Print and shaded views of the part. All mm, measured from the part's lowest x, y and z. A direction names the side the tool comes from. Round coordinates to 2 decimals unless told otherwise and drop trailing zeros. Order: outer loops, then holes, each group sorted by start corner. A loop starts at its lowest first (then second) coordinate and runs counter-clockwise, first axis right, second up. Notation, with made-up numbers: M 62.5,-28 L 94.5,-28 A14 ccw 94.5,-2 Z; hole C 26.5,13 d3. An arc over 180 degrees is marked long. Write each question's results on one line, items separated by ' | '. Start each with the question number.
1. Probe L1, parallel to X at y = 1.5, z = 9.75; L2, parallel to Y at x = 62.5, z = 9.5; L3, parallel to Y at x = 62.5, z = 17.75. List the from-to ranges inside material, lowest first. Write a range as [from, to].
2. Which spindle directions (+Z, -Z, +X, -X, +Y, -Y) get a long thin tool onto all of the face, cutting with end or side? Do the marked faces 4, 5 and 6. Say none if no direction does.
3. Drop flat-ended pins along their axis: pin 1 Ø3 at (x, z) = (30.5, 6.5) entering from -Y; pin 2 Ø2 at (y, z) = (11.5, 17.5) entering from -X; pin 3 Ø12 at (x, y) = (45.5, 4.5) entering from -Z. Give the stop position or say it passes through.
4. Band-saw the part on B-B, the plane y = 1. List the corners of the cut face in (x, z), then the cut area to 3 significant figures.
5. Band-saw the part on C-C, the plane x = 76. List the corners of the cut face in (y, z), then the cut area to 3 significant figures.
6. Two-plate mould, pull along X, no slides. Class the marked faces 1, 2 and 3: +X half, -X half, draft (parallel to the pull), parting line (faces both ways), or undercut.
7. Band-saw the part on A-A, the plane z = 17. List the corners of the cut face in (x, y).
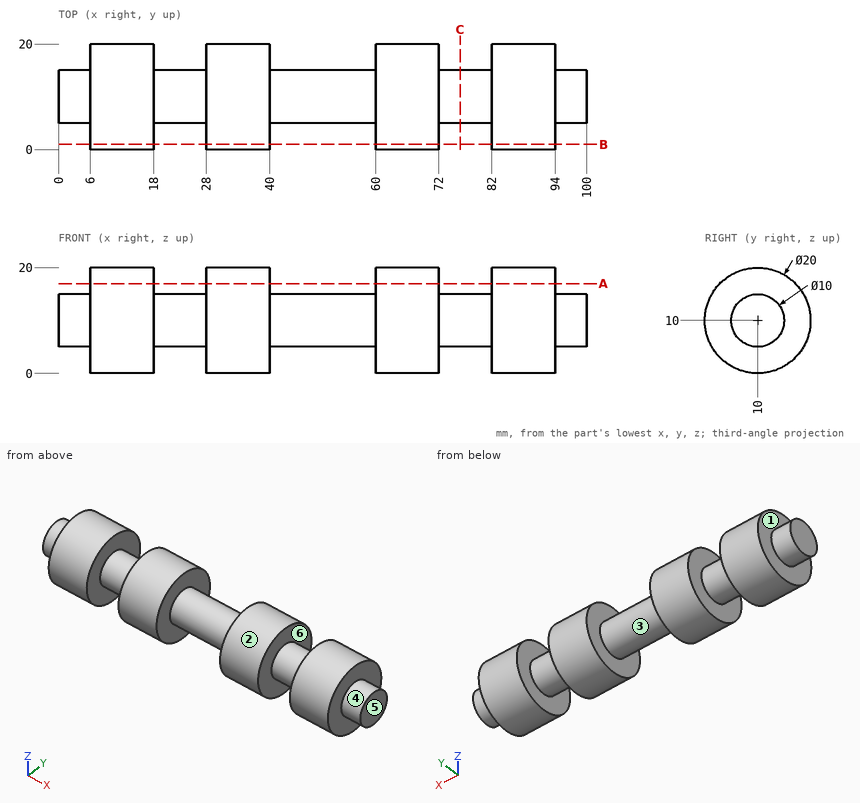
Solution:
1) L1: [6, 18], [28, 40], [60, 72], [82, 94] | L2: [0.01, 19.99] | L3: [3.68, 16.32]
2) face 4: +X | face 5: +Z, -Z, +X, +Y, -Y | face 6: none
3) pin 1: y = 0.2 | pin 2: x = 6 | pin 3: z = 0.49
4) outline: M 6,5.64 L 18,5.64 L 18,14.36 L 6,14.36 Z; M 28,5.64 L 40,5.64 L 40,14.36 L 28,14.36 Z; M 60,5.64 L 72,5.64 L 72,14.36 L 60,14.36 Z; M 82,5.64 L 94,5.64 L 94,14.36 L 82,14.36 Z | area: 418 mm^2
5) outline: C 10,10 d10 | area: 78.5 mm^2
6) face 1: -X half | face 2: draft | face 3: undercut
7) outline: M 6,2.86 L 18,2.86 L 18,17.14 L 6,17.14 Z; M 28,2.86 L 40,2.86 L 40,17.14 L 28,17.14 Z; M 60,2.86 L 72,2.86 L 72,17.14 L 60,17.14 Z; M 82,2.86 L 94,2.86 L 94,17.14 L 82,17.14 Z
